Can you work these out from the model? Positions are in its coordinate system, mm. Face numbers are marked on the shaded views. A direction names the side the tool comes from. Give positions to 0.01 mm unless a question says otherwise; leave off trailing zeros. Order: outer loops, then holes, each group sorted by start corner. A loop starts at its lowest first (then second) coordinate and runs counter-clockwise, first axis right, second up.
Item 1: I want a section at D-D, the plane x = -30. Write out the boundary of the cut face in (y, z), then the cut area to 3 significant figures.
Item 2: I'm going to push flat-ended pins straight in: pin 1 Ø12 at (x, z) = (-45, 16.5) entering from -Y; pin 2 Ø2 at (x, y) = (-18.5, -19) entering from -Z; pin 3 Ø10 at (x, z) = (17.5, 29) entering from +Y; pin 4 Ø6 at (x, z) = (-21, 18) entering from +Y. Where does each tip first touch, or does it pass through?
Item 3: I want a section at C-C, the plane z = 20. Write out the boundary of the cut face in (x, y), then the cut area to 3 significant figures.
Item 4: I want a section at A-A, the plane x = 9.5. Write out the boundary of the cut face in (y, z), then the cut area to 3 significant figures.
Item 5: If I drill on line 1 along Z through (x, y) = (54, -35); line 2 along X through (y, z) = (52.5, 9.5); line 3 along X through (y, z) = (-47, 28), over which ranges is the centre line in solid material (lowest first)?
Item 6: If we mould it in two halves opening along Y, with no side actions, what happens to the marked faces 1, 2 and 3? For each: +Y half, -Y half, draft (parallel to the pull), parting line (faces both ways), or undercut.
Item 7: Which directions (+Z, -Z, +X, -X, +Y, -Y) give clear straight access to the entire face, cutting with the end or side of a thin tool? Please do the marked faces 4 and 5.
Item 8: I want a section at B-B, the plane y = -23. Write out the boundary of the cut face in (x, z).
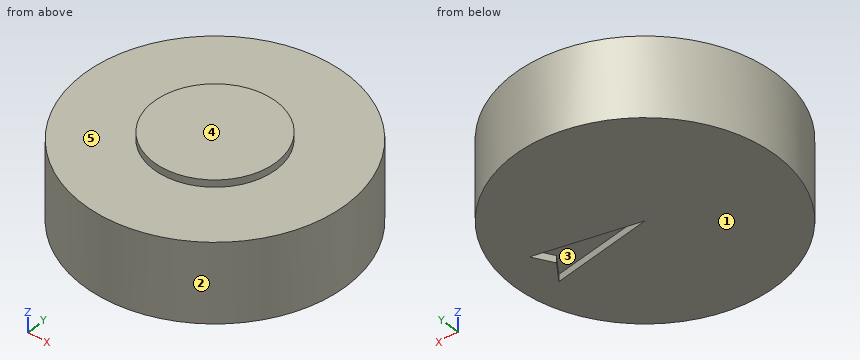
```python
from build123d import *

# Parameters (mm, degrees)
SKETCH_1_R          = 74
EXTRUDE_1_DEPTH     = 44.8
SKETCH_3_R          = 34.5
EXTRUDE_2_DEPTH     = 4
CUT_EXTRUDE_3_DEPTH = 4


with BuildPart() as part:
    # 草图1 → 凸台-拉伸1 (new body)
    with BuildSketch(Plane.XY):
        Circle(SKETCH_1_R)
    extrude(amount=EXTRUDE_1_DEPTH)

    # 草图3 → 凸台-拉伸2 (add)
    with BuildSketch(Plane.XY.offset(44.8)):
        Circle(SKETCH_3_R)
    extrude(amount=EXTRUDE_2_DEPTH)

    # 草图4 → 切除-拉伸3 (cut)
    with BuildSketch(Plane(origin=(0, 0, 0), x_dir=(1, 0, 0), z_dir=(0, 0, -1))):
        Polygon((55.454566514, -11.572321894), (0, 0), (56.650713471, 10.308727493), (48.957646125, -0.806969816), align=None)
    extrude(amount=-CUT_EXTRUDE_3_DEPTH, mode=Mode.SUBTRACT)


solid = part.part
```
Results list:
1. outline: (-67.65, 0) - (67.65, 0) - (67.65, 44.8) - (17.04, 44.8) - (17.04, 48.8) - (-17.04, 48.8) - (-17.04, 44.8) - (-67.65, 44.8) - close
1. area: 6,200 mm2
2. pin 1: stops at y = -62.89
2. pin 2: stops at z = 0
2. pin 3: stops at y = 72.94
2. pin 4: stops at y = 71.78
3. outline: circle Ø148 at (0, 0)
3. area: 17,200 mm2
4. outline: (-73.39, 0) - (-1.73, 0) - (-1.73, 4) - (1.98, 4) - (1.98, 0) - (73.39, 0) - (73.39, 44.8) - (33.17, 44.8) - (33.17, 48.8) - (-33.17, 48.8) - (-33.17, 44.8) - (-73.39, 44.8) - close
4. area: 6,830 mm2
5. line 1: z = 0 to 44.8
5. line 2: x = -52.15 to 52.15
5. line 3: x = -57.16 to 57.16
6. face 1: draft
6. face 2: parting line
6. face 3: undercut
7. face 4: +Z, +X, -X, +Y, -Y
7. face 5: +Z
8. outline: (-70.33, 0) - (70.33, 0) - (70.33, 44.8) - (25.71, 44.8) - (25.71, 48.8) - (-25.71, 48.8) - (-25.71, 44.8) - (-70.33, 44.8) - close
